The model under review builds one solid part; all positions refer to its coordinate system, in mm. Round coordinates to 2 decimals unless told otherwise and drop trailing zeros. Order: outer loops, then holes, each group sorted by start corner. A loop starts at its lowest first (then second) coordinate and runs counter-clockwise, first axis right, second up. Notation, with made-up numbers: (7, 79) - (52, 79) arc R25 ccw to (52, 103) - close; hole circle Ø6 at (24.25, -34.75). An arc over 180 degrees is marked (long way). One line per question, with ' | ' between items. Start each with the question number.
Item 1: Add section B-B on y = 51.3. State the section outline as (x, z) points, and give its area (3 significant figures).
Item 2: For L1, parallel to Y at x = 1.5, z = 1.5; L2, parallel to Y at x = 17.5, z = 1.1; L3, parallel to X at y = -14, z = 0.5, list the stretches that pass through material, from the lowest coordinate up. Write a range as [from, to].
Item 3: Add section D-D on y = 4. State the section outline as (x, z) points, and give its area (3 significant figures).
Item 4: Add section A-A on x = 1.5. State the section outline as (y, z) points, and give its area (3 significant figures).
Item 5: Add section C-C on z = 1.15. State the section outline as (x, y) points.
Item 6: Draft analysis for pull direction X (two halves, no side actions). For faces 1 (the face through (19.9, -17.13, 1.01)), 2 (the face through (8.22, 46.84, 1.01)), 3 (the face through (-16.93, -17.1, 1.01)), state which applies: +X half, -X half, draft (parallel to the pull), parting line (faces both ways), or undercut.
from build123d import *

# Parameters (mm, degrees)
SKETCH1_W           = 38
SKETCH1_H           = 72
SKETCH1_R           = 1.6
BOSS_EXTRUDE1_DEPTH = 2
SKETCH2_R           = 12.5
CUT_EXTRUDE1_DEPTH  = 59.075295953
FILLET2_R           = 2


with BuildPart() as part:
    # Sketch1 → Boss-Extrude1 (new body)
    with BuildSketch(Plane.XY):
        with Locations((1.5, 18.3)):
            Rectangle(SKETCH1_W, SKETCH1_H)
        with Locations((17.5, -14.7)):
            Circle(SKETCH1_R, mode=Mode.SUBTRACT)
        with Locations((-14.5, -14.7)):
            Circle(SKETCH1_R, mode=Mode.SUBTRACT)
        with Locations((17.5, 51.3)):
            Circle(SKETCH1_R, mode=Mode.SUBTRACT)
        with Locations((-14.5, 51.3)):
            Circle(SKETCH1_R, mode=Mode.SUBTRACT)
    extrude(amount=BOSS_EXTRUDE1_DEPTH)

    # Sketch2 → Cut-Extrude1 (cut, through all)
    with BuildSketch(Plane.XY.offset(2)):
        with Locations((1.5, 0.3)):
            Circle(SKETCH2_R)
        with Locations((1.5, 36.3)):
            Circle(SKETCH2_R)
    extrude(amount=-CUT_EXTRUDE1_DEPTH, mode=Mode.SUBTRACT)

    # Fillet2
    fillet2_edges = [part.edges().sort_by_distance(p)[0] for p in [
        (20.5, -17.7, 1),
        (-17.5, -17.7, 1),
        (-17.5, 54.3, 1),
        (20.5, 54.3, 1),
    ]]
    fillet(fillet2_edges, radius=FILLET2_R)


solid = part.part
Determined:
1) outline: (-17.5, 0) - (-16.1, 0) - (-16.1, 2) - (-17.5, 2) - close; (-12.9, 0) - (15.9, 0) - (15.9, 2) - (-12.9, 2) - close; (19.1, 0) - (20.5, 0) - (20.5, 2) - (19.1, 2) - close | area: 63.2 mm2
2) L1: [-17.7, -12.2], [12.8, 23.8], [48.8, 54.3] | L2: [-17.7, -16.3], [-13.1, 49.7], [52.9, 54.3] | L3: [-17.5, -15.94], [-13.06, 16.06], [18.94, 20.5]
3) outline: (-17.5, 0) - (-10.44, 0) - (-10.44, 2) - (-17.5, 2) - close; (13.44, 0) - (20.5, 0) - (20.5, 2) - (13.44, 2) - close | area: 28.2 mm2
4) outline: (-17.7, 0) - (-12.2, 0) - (-12.2, 2) - (-17.7, 2) - close; (12.8, 0) - (23.8, 0) - (23.8, 2) - (12.8, 2) - close; (48.8, 0) - (54.3, 0) - (54.3, 2) - (48.8, 2) - close | area: 44.0 mm2
5) outline: (-17.5, -15.7) arc R2 ccw to (-15.5, -17.7) - (18.5, -17.7) arc R2 ccw to (20.5, -15.7) - (20.5, 52.3) arc R2 ccw to (18.5, 54.3) - (-15.5, 54.3) arc R2 ccw to (-17.5, 52.3) - close; hole circle Ø3.2 at (-14.5, -14.7); hole circle Ø3.2 at (-14.5, 51.3); hole circle Ø25 at (1.5, 0.3); hole circle Ø25 at (1.5, 36.3); hole circle Ø3.2 at (17.5, -14.7); hole circle Ø3.2 at (17.5, 51.3)
6) face 1: +X half | face 2: undercut | face 3: -X half
